Autodesk Inventor part; units mm, degrees
ref_plane "YZ Plane" through (0, 0, 0) normal (1, 0, 0) x (0, 1, 0)
ref_plane "XZ Plane" through (0, 0, 0) normal (0, 1, 0) x (-1, 0, 0)
ref_plane "XY Plane" through (0, 0, 0) normal (0, 0, 1) x (1, 0, 0)
sketch "Sketch1" plane through (0, 0, 0) normal (0, 1, 0) x (-1, 0, 0)
  line L0 (0, 0) -> (50.8, 0)
  line L1 (50.8, 0) -> (50.8, 254)
  line L2 (50.8, 254) -> (0, 254)
  line L3 (0, 254) -> (0, 0)
  dimension "d0" = 50.8
  dimension "d1" = 254
extrude "Extrusion1" add sketch "Sketch1" along normal blind 6.35
sketch "Sketch2" plane through (0, 6.35, 0) normal (0, 1, 0) x (1, 0, 0)
  line L0 (-50.8, -254) -> (0, -254)
  circle A0 centre (-25.4, -228.6) radius 6.9766
  dimension "d4" = 25.4
extrude "Extrusion2" cut sketch "Sketch2" against normal blind 25.4
properties part number "heightMarker" material "Gold"
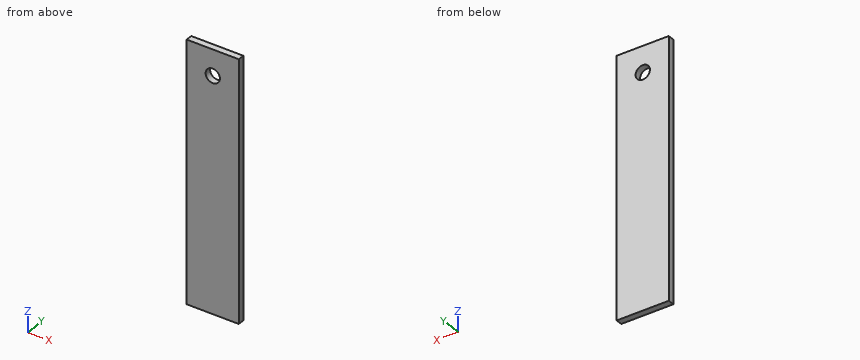
Model file for the job. Use its own axes, mm. Give positions to 0.01 mm unless a question says otherwise; leave off trailing zeros. Order: outer loops, then holes, each group sorted by start corner. A loop starts at its lowest first (then second) coordinate and runs counter-clockwise, first axis right, second up. Notation, with made-up numbers: M -35,15.25 L 7,15.25 A5 ccw 7,20.25 Z; hole C 32,78.25 d10. An arc over 180 degrees is marked long. Put each result on its own line as item: value. Start each with the question number.
(1) Drill centre lines: L1, parallel to Z at x = -25.4, y = 2.5; L2, parallel to X at y = 4.5, z = 228.6; L3, parallel to X at y = 1, z = 235. Where is each one in solid material? Low to high. Write a range as [from, to].
(2) Pin check, flat tip, straight feed: pin 1 Ø11 at (x, z) = (-25.4, 228.6) entering from -Y (3 decimals). Stop position of the tip, or through.
(3) Band-saw the part on B-B on x = -25.4. Give the cut face in (y, z), then the cut area to 3 significant figures.
(4) Band-saw the part on A-A on z = 228.6. Give the cut face in (x, y), then the cut area to 3 significant figures.
Results below:
1. L1: z = [0, 221.62], [235.58, 254]
1. L2: x = [-50.8, -32.38], [-18.42, 0]
1. L3: x = [-50.8, -28.18], [-22.62, 0]
2. pin 1: passes through
3. outline: M 0,0 L 6.35,0 L 6.35,221.62 L 0,221.62 Z; M 0,235.58 L 6.35,235.58 L 6.35,254 L 0,254 Z
3. area: 1,520 mm2
4. outline: M -50.8,0 L -32.38,0 L -32.38,6.35 L -50.8,6.35 Z; M -18.42,0 L 0,0 L 0,6.35 L -18.42,6.35 Z
4. area: 234 mm2
